Part model, mm, in its own coordinate system. Round coordinates to 2 decimals unless told otherwise and drop trailing zeros.
1) Probe line 1 (Y direction, x = 647.7, z = 1.35); line 2 (Y direction, x = 939.8, z = 1.75); line 3 (Y direction, x = 639, z = 0.5). List the from-to ranges inside material, lowest first.
2) Drop flat-ended pins along their axis: P1, Ø5, axis at x = 1053.66, y = 762, coming from the +Z side; P2, Ø8, axis at x = 279.4, y = 432.3, coming from the -Z side; P3, Ø11.5, axis at x = 647.7, y = 432.4, coming from the +Z side. Give the stop position or say it passes through.
3) Band-saw the part on A-A, the plane z = 1.25. State how many separate pieces and enclosed holes the cut face has, then the cut area to 3 significant figures.
from build123d import *

# Parameters (mm, degrees)
SKETCH1_W                                     = 1219.2
SKETCH1_H                                     = 1981.2
SKETCH1_W_2                                   = 863.6
SKETCH1_H_2                                   = 254
BOSS_EXTRUDE1_DEPTH                           = 6.35
CSK_FOR_1_4_FLAT_HEAD_MACHINE_SCREW1_AT_COUNT = 2
CSK_FOR_1_4_FLAT_HEAD_MACHINE_SCREW1_AT_PITCH = 76.2
CSK_FOR_1_4_FLAT_HEAD_MACHINE_SCREW1_2_COUNT  = 2
CSK_FOR_1_4_FLAT_HEAD_MACHINE_SCREW1_2_PITCH  = 736.600036601
CSK_FOR_1_4_FLAT_HEAD_MACHINE_SCREW1_3_COUNT  = 2
CSK_FOR_1_4_FLAT_HEAD_MACHINE_SCREW1_3_PITCH  = 812.800033169
CSK_FOR_1_4_FLAT_HEAD_MACHINE_SCREW1_4_COUNT  = 2
CSK_FOR_1_4_FLAT_HEAD_MACHINE_SCREW1_4_PITCH  = 368.300013149
CSK_FOR_1_4_FLAT_HEAD_MACHINE_SCREW1_5_COUNT  = 2
CSK_FOR_1_4_FLAT_HEAD_MACHINE_SCREW1_5_PITCH  = 444.500010895
FILLET1_R                                     = 3.175
F_5_16_0_3125_DIAMETER_HOLE2_D                = 7.9375


with BuildPart() as part:
    # Sketch1 → Boss-Extrude1 (new body)
    with BuildSketch(Plane.XY):
        with Locations((609.6, 990.6)):
            Rectangle(SKETCH1_W, SKETCH1_H)
        with Locations((609.6, 584.2)):
            Rectangle(SKETCH1_W_2, SKETCH1_H_2, mode=Mode.SUBTRACT)
    extrude(amount=BOSS_EXTRUDE1_DEPTH)

    # Sketch3 → CSK for 1/4 Flat Head Machine Screw1 (revolve, cut)
    with BuildSketch(Plane(origin=(203.2, 432.304928843, 6.35), x_dir=(0, -1, 0), z_dir=(1, 0, 0))):
        Polygon((0, 0), (0, 6.35), (3.57124, 6.35), (3.57124, 3.298865467), (6.4389, 0), align=None)
    csk_for_1_4_flat_head_machine_screw1 = revolve(axis=Axis((203.2, 432.304928843, 12.7), (0, 0, -1)), mode=Mode.SUBTRACT)

    # CSK for 1/4 Flat Head Machine Screw1 at: CSK for 1/4 Flat Head Machine Screw1 ×2
    with Locations(*[(i * CSK_FOR_1_4_FLAT_HEAD_MACHINE_SCREW1_AT_PITCH, 0, 0) for i in range(1, CSK_FOR_1_4_FLAT_HEAD_MACHINE_SCREW1_AT_COUNT)]):
        add(csk_for_1_4_flat_head_machine_screw1, mode=Mode.SUBTRACT)

    # CSK for 1_4 Flat Head Machine Screw1 2: CSK for 1/4 Flat Head Machine Screw1 ×2
    with Locations(*[Vector(0.99999995, 0.000315241, 0) * (i * CSK_FOR_1_4_FLAT_HEAD_MACHINE_SCREW1_2_PITCH) for i in range(1, CSK_FOR_1_4_FLAT_HEAD_MACHINE_SCREW1_2_COUNT)]):
        add(csk_for_1_4_flat_head_machine_screw1, mode=Mode.SUBTRACT)

    # CSK for 1_4 Flat Head Machine Screw1 3: CSK for 1/4 Flat Head Machine Screw1 ×2
    with Locations(*[Vector(0.999999959, 0.000285687, 0) * (i * CSK_FOR_1_4_FLAT_HEAD_MACHINE_SCREW1_3_PITCH) for i in range(1, CSK_FOR_1_4_FLAT_HEAD_MACHINE_SCREW1_3_COUNT)]):
        add(csk_for_1_4_flat_head_machine_screw1, mode=Mode.SUBTRACT)

    # CSK for 1_4 Flat Head Machine Screw1 4: CSK for 1/4 Flat Head Machine Screw1 ×2
    with Locations(*[Vector(0.999999964, 0.000267211, 0) * (i * CSK_FOR_1_4_FLAT_HEAD_MACHINE_SCREW1_4_PITCH) for i in range(1, CSK_FOR_1_4_FLAT_HEAD_MACHINE_SCREW1_4_COUNT)]):
        add(csk_for_1_4_flat_head_machine_screw1, mode=Mode.SUBTRACT)

    # CSK for 1_4 Flat Head Machine Screw1 5: CSK for 1/4 Flat Head Machine Screw1 ×2
    with Locations(*[Vector(0.999999975, 0.000221404, 0) * (i * CSK_FOR_1_4_FLAT_HEAD_MACHINE_SCREW1_5_PITCH) for i in range(1, CSK_FOR_1_4_FLAT_HEAD_MACHINE_SCREW1_5_COUNT)]):
        add(csk_for_1_4_flat_head_machine_screw1, mode=Mode.SUBTRACT)

    # Fillet1
    fillet1_edges = [part.edges().sort_by_distance(p)[0] for p in [
        (177.8, 711.2, 3.175),
        (177.8, 457.2, 3.175),
        (1041.4, 457.2, 3.175),
        (1041.4, 711.2, 3.175),
        (0, 1981.2, 3.175),
        (1219.2, 1981.2, 3.175),
        (1219.2, 0, 3.175),
        (0, 0, 3.175),
    ]]
    fillet(fillet1_edges, radius=FILLET1_R)

    # 5/16 (0.3125) Diameter Hole2 (through all)
    with Locations(Plane.XY.offset(6.35)):
        with Locations((609.6, 938.2125), (111.5695, 762), (111.5695, 152.4), (165.5445, 152.4), (165.5445, 762), (1053.6555, 152.4), (1107.6305, 152.4), (1107.6305, 762), (1053.6555, 762), (609.6, 884.2375)):
            Hole(F_5_16_0_3125_DIAMETER_HOLE2_D / 2)


solid = part.part
Reported:
1. line 1: y = 0 to 428.83, 435.97 to 457.2, 711.2 to 1981.2
1. line 2: y = 0 to 428.97, 436.11 to 457.2, 711.2 to 1981.2
1. line 3: y = 0 to 457.2, 711.2 to 1981.2
2. P1: passes through
2. P2: stops at z = 0
2. P3: stops at z = 5.56
3. separate pieces: 1
3. enclosed holes: 17
3. area: 2,200,000 mm2
